Can you work these out from the model? Positions are in its coordinate system, mm. A direction names the side the tool comes from. Give positions to 0.01 mm unless a question says otherwise; leave off trailing zeros. Write each loop counter-clockwise with the first axis right and the second up, starting at its lowest first coordinate (ties: lowest second). Pieces come first, ordered by that corner, then holes. Notation, with made-up numbers: (37.5, 79.25) - (43.5, 79.25) arc R18 ccw to (43.5, 86.25) - close; hole circle Ø6 at (-34, 63). An arc over 180 degrees is marked (long way). Use a Markdown table: item, result. Add a question column.
```python
from build123d import *

# Parameters (mm, degrees)
CHAMFER1_SIZE = 1


with BuildPart() as part:
    # Sketch1 → Revolve1 (revolve)
    with BuildSketch(Plane.XY):
        Polygon((0, 1.9), (0, 5), (-48, 5), (-48, 0), (-4, 0), (-3.248924226, 1.25), (-1.125833025, 1.25), align=None)
    revolve(axis=Axis((0, 0, 0), (-1, 0, 0)))

    # Chamfer1
    chamfer1_edges = [part.edges().sort_by_distance(p)[0] for p in [
        (0, -5, 0),
        (-48, -5, 0),
    ]]
    chamfer(chamfer1_edges, length=CHAMFER1_SIZE)


solid = part.part
```
Q1. I'm going to push a flat-ended pin straight in: P1, Ø1.5, axis at x = -21, z = -1, coming from the -Y side. Where does the tip first touch, or does it pass through?
Q2. On a 3-axis mill with a long thin cutter (end or side, diameter ignored), from which of +Z, -Z, +X, -X, +Y, -Y can I reach the whole of each face in a straight line? I mean faces 4 (the cylindrical face through (-2.17, -0.27, 1.22)), 5 (the flat face through (0, -2, 1)). Say none if no direction works.
Q3. If we mould it in two halves opening along Z, with no side actions, what happens to faces 1 (the cylindrical face through (-24.32, -1.08, 4.88)), 2 (the flat face through (-48, 0, 0)), 3 (the conical face through (-4, 0, 0))? For each: released by +Z, released by -Z, zero draft, split by the parting line, or undercut.
Q4. Suppose I cut it at A-A (x = -6). Please give me the cut outline in (y, z).
Q5. If I drill on probe 1 along Z at (x, y) = (-1.55, 0); probe 2 along Z at (x, y) = (-6, 2), over which ranges is the centre line in solid material (lowest first)? Write a range as [from, to].
Derived:
| question | item | result |
|---|---|---|
| 1 | P1 | y = -4.99 |
| 2 | face 4 | +X |
| 2 | face 5 | +Z, -Z, +X, +Y, -Y |
| 3 | face 1 | split by the parting line |
| 3 | face 2 | zero draft |
| 3 | face 3 | undercut |
| 4 | outline | circle Ø10 at (0, 0) |
| 5 | probe 1 | [-5, -1.25], [1.25, 5] |
| 5 | probe 2 | [-4.58, 4.58] |
